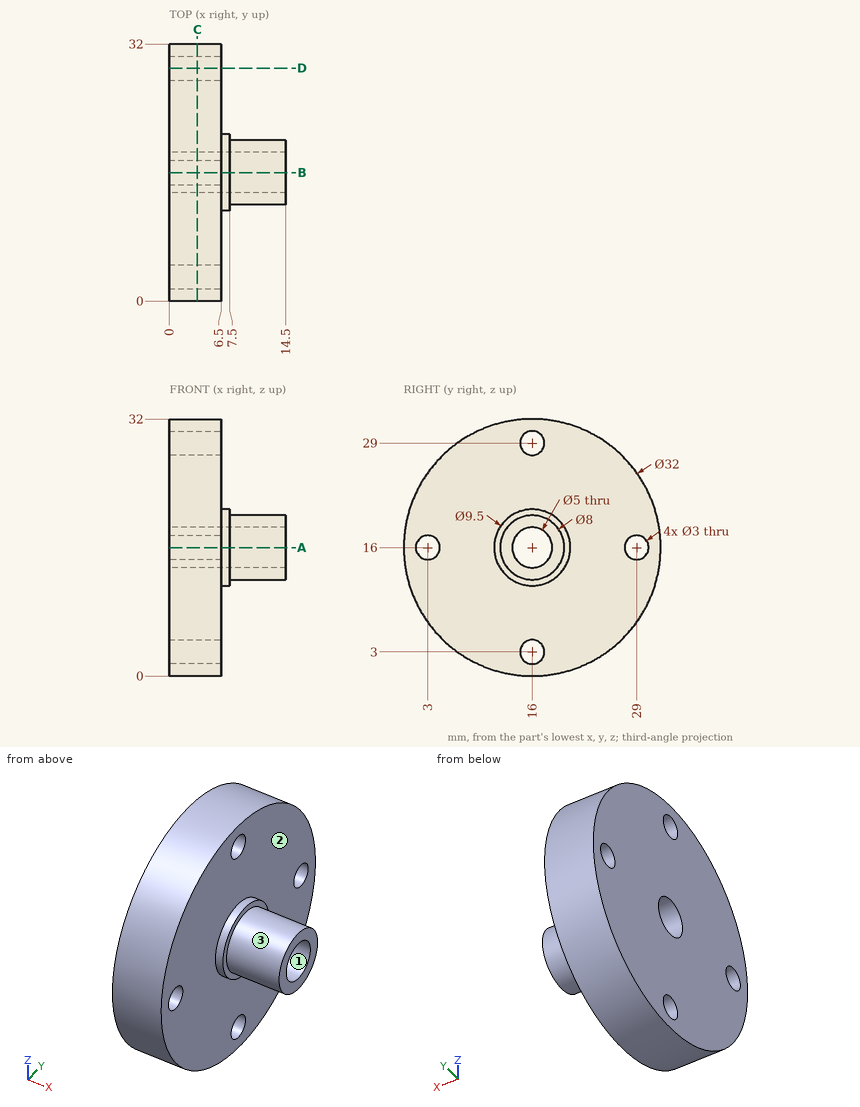
Here's the drawing with two shaded views (mm, measured from the low corner). I have some questions. Round coordinates to 2 decimals unless told otherwise and drop trailing zeros. Order: outer loops, then holes, each group sorted by start corner. A loop starts at its lowest first (then second) coordinate and runs counter-clockwise, first axis right, second up. Notation, with made-up numbers: (85.5, -36.5) -> (116.5, -36.5) arc R27 cw to (116.5, -13.5) -> close; hole circle Ø7 at (-12.75, -25.75). An arc over 180 degrees is marked (long way). Return JSON: item names as keys, results as strings.
Q1. If we section it at D-D on y = 29: List the corners of the cut face in (x, z) for me, plus the area to 3 significant figures.
Filled sheet:
{"outline": "(0, 6.67) -> (6.5, 6.67) -> (6.5, 14.5) -> (0, 14.5) -> close; (0, 17.5) -> (6.5, 17.5) -> (6.5, 25.33) -> (0, 25.33) -> close", "area": "102 mm^2"}
Q2. I need wall thicknesses on line 1 along Y through (x, z) = (4.5, 16); line 2 along X through (y, z) = (9.5, 6); line 3 along X through (y, z) = (20.5, 17). Which ranges of each line are inside material? Lowest first, please. Write a range as from..to.
Filled sheet:
{"line 1": "y = 0..1.5, 4.5..13.5, 18.5..27.5, 30.5..32", "line 2": "x = 0..6.5", "line 3": "x = 0..7.5"}
Q3. For pin 1 Ø2.5 at (y, z) = (16, 3) entering from -X; pin 2 Ø6 at (y, z) = (24.5, 6.5) entering from +X; pin 3 Ø6 at (x, y) = (10.5, 10) entering from +Z; pin 4 Ø1.5 at (x, y) = (1.5, 14.5) entering from -Z, each with a flat end and sliding along its axis, tell me the tip position at first contact or that it passes through.
Filled sheet:
{"pin 1": "passes through", "pin 2": "stops at x = 6.5", "pin 3": "stops at z = 18.65", "pin 4": "stops at z = 0.02"}
Q4. If we mould it in two halves opening along Z, with no side actions, what happens to the marked faces 1, 2 and 3? For each: released by +Z, released by -Z, zero draft, split by the parting line, or undercut.
Filled sheet:
{"face 1": "undercut", "face 2": "zero draft", "face 3": "split by the parting line"}
Q5. If we section it at A-A on z = 16: List the corners of the cut face in (x, y) for me, plus the area to 3 significant figures.
Filled sheet:
{"outline": "(0, 0) -> (6.5, 0) -> (6.5, 1.5) -> (0, 1.5) -> close; (0, 4.5) -> (6.5, 4.5) -> (6.5, 11.25) -> (7.5, 11.25) -> (7.5, 12) -> (14.5, 12) -> (14.5, 13.5) -> (0, 13.5) -> close; (0, 18.5) -> (14.5, 18.5) -> (14.5, 20) -> (7.5, 20) -> (7.5, 20.75) -> (6.5, 20.75) -> (6.5, 27.5) -> (0, 27.5) -> close; (0, 30.5) -> (6.5, 30.5) -> (6.5, 32) -> (0, 32) -> close", "area": "162 mm^2"}
Q6. If we section it at C-C on x = 3.5: List the corners of the cut face in (y, z) for me.
Filled sheet:
{"outline": "circle Ø32 at (16, 16); hole circle Ø3 at (3, 16); hole circle Ø5 at (16, 16); hole circle Ø3 at (16, 3); hole circle Ø3 at (16, 29); hole circle Ø3 at (29, 16)"}
